Can you work these out from the drawing? Everything is in mm from the part's minimum corner. Round coordinates to 2 decimals unless told otherwise and drop trailing zeros. Write each loop counter-clockwise with the first axis right and the second up, starting at its lowest first coordinate (ties: lowest second). Pieces come first, ordered by that corner, then holes. Notation, with made-up numbers: (39, 3.25) -> (67, 3.25) arc R30 ccw to (67, 35.25) -> close; hole circle Ø5 at (52.5, 20). An arc over 180 degrees is marked (long way). Write item = value, one per line. Start each with the question number.
1) If I drill on line 1 (X direction, y = 0.7, z = 3.5); line 2 (Z direction, x = 32, y = 0.9); line 3 (Z direction, x = 3, y = 0.4), over which ranges is the centre line in solid material (lowest first)?
2) Imagine slicing it at C-C, the plane y = 2.55. Please give me the cut outline in (x, z).
3) Imagine slicing it at D-D, the plane x = 15. Please give me the cut outline in (y, z).
4) I'm going to push a flat-ended pin straight in: pin 1 (3 mm diameter, centred on x = 3.5, z = 3.5, fed in from -Y). Where does the tip first touch, or does it pass through?
5) Imagine slicing it at A-A, the plane z = 3.5. Please give me the cut outline in (x, y), then the cut area to 3 significant figures.
6) Imagine slicing it at B-B, the plane x = 3.5. Please give me the cut outline in (y, z).
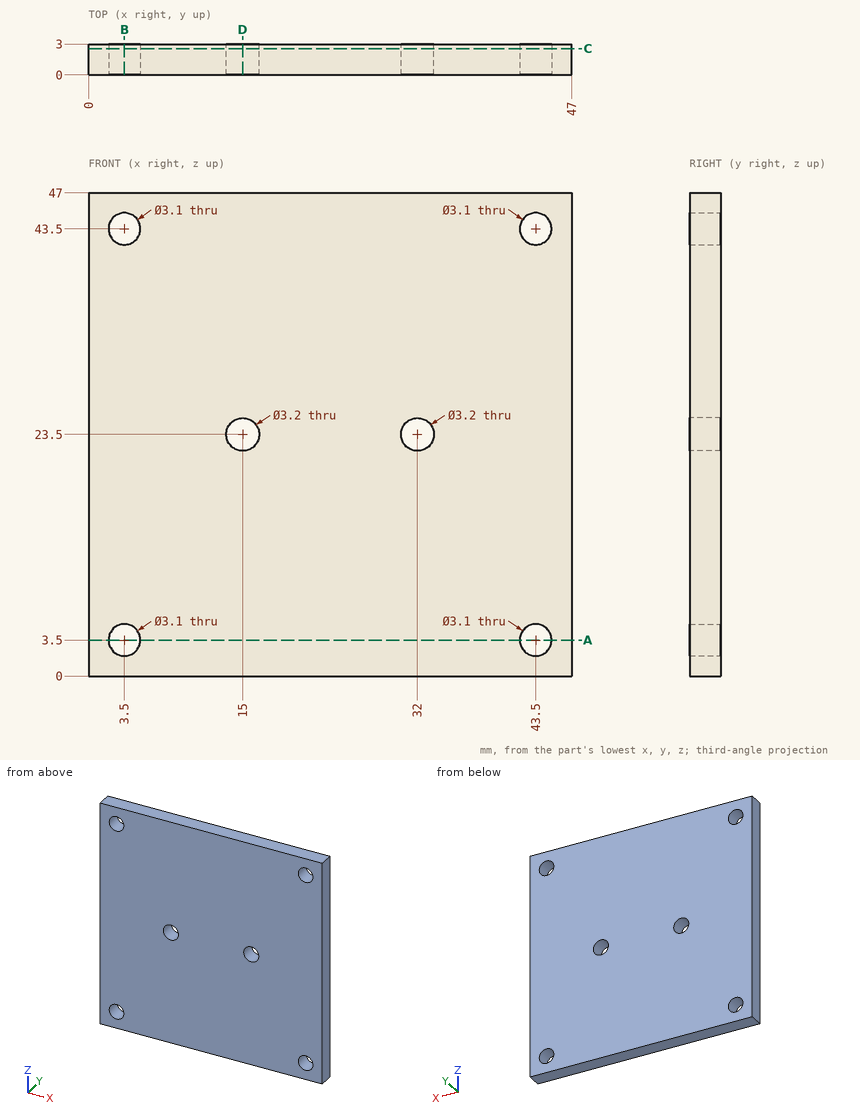
Reported:
q1.line_1 = 0 to 1.95, 5.05 to 41.95, 45.05 to 47
q1.line_2 = 0 to 21.9, 25.1 to 47
q1.line_3 = 0 to 2.03, 4.97 to 42.03, 44.97 to 47
q2.outline = (0, 0) -> (47, 0) -> (47, 47) -> (0, 47) -> close; hole circle Ø3.1 at (3.5, 3.5); hole circle Ø3.1 at (3.5, 43.5); hole circle Ø3.2 at (15, 23.5); hole circle Ø3.2 at (32, 23.5); hole circle Ø3.1 at (43.5, 3.5); hole circle Ø3.1 at (43.5, 43.5)
q3.outline = (0, 0) -> (3, 0) -> (3, 21.9) -> (0, 21.9) -> close; (0, 25.1) -> (3, 25.1) -> (3, 47) -> (0, 47) -> close
q4.pin_1 = through
q5.outline = (0, 0) -> (1.95, 0) -> (1.95, 3) -> (0, 3) -> close; (5.05, 0) -> (41.95, 0) -> (41.95, 3) -> (5.05, 3) -> close; (45.05, 0) -> (47, 0) -> (47, 3) -> (45.05, 3) -> close
q5.area = 122 mm²
q6.outline = (0, 0) -> (3, 0) -> (3, 1.95) -> (0, 1.95) -> close; (0, 5.05) -> (3, 5.05) -> (3, 41.95) -> (0, 41.95) -> close; (0, 45.05) -> (3, 45.05) -> (3, 47) -> (0, 47) -> close
